Part model, mm, in its own coordinate system. Face numbers are marked on the shaded views. A direction names the side the tool comes from. Round coordinates to 2 decimals unless told otherwise and drop trailing zeros. Loops run counter-clockwise (first coordinate to the right, second up) from the corner with the lowest first, then second, coordinate; pieces in that order, holes last. Notation, with made-up numbers: M 86,84 L 101,84 A15 ccw 101,106 Z; hole C 46,58.25 d2. An arc over 180 degrees is marked long. Answer as CSV lines item,"result". Start each with the question number.
Item 1: Which spindle directions (+Z, -Z, +X, -X, +Y, -Y) get a long thin tool onto all of the face, cutting with end or side? Do the marked faces 1 and 2. Say none if no direction does.
Item 2: Mould opens along X. For the marked faces 3, 4 and 5 say: pulls with the +X half, pulls with the -X half, needs draft (parallel to the pull), parting line crosses it, or undercut.
Item 3: Drop flat-ended pins along their axis: pin 1 Ø2 at (y, z) = (28, -23.5) entering from -X; pin 2 Ø2 at (x, z) = (-12, -23.5) entering from -Y; pin 3 Ø2.5 at (x, y) = (-16, 5) entering from -Z. Give the stop position or say it passes through.
Item 4: Band-saw the part on A-A (x = 0). Give the cut face in (y, z), and give its area (3 significant figures).
Item 5: Band-saw the part on D-D (z = -17). Give the cut face in (x, y).
Item 6: Wall check: line 1 (X direction, y = 53.5, z = -8.5); line 2 (Y direction, x = 5, z = -29.5); line 3 (Z direction, x = -15.55, y = 0). Give the ranges that are in metal, low to high.
Item 7: Band-saw the part on B-B (z = 0). Give the cut face in (x, y).
Item 8: Band-saw the part on C-C (y = 46). Give the cut face in (x, z).
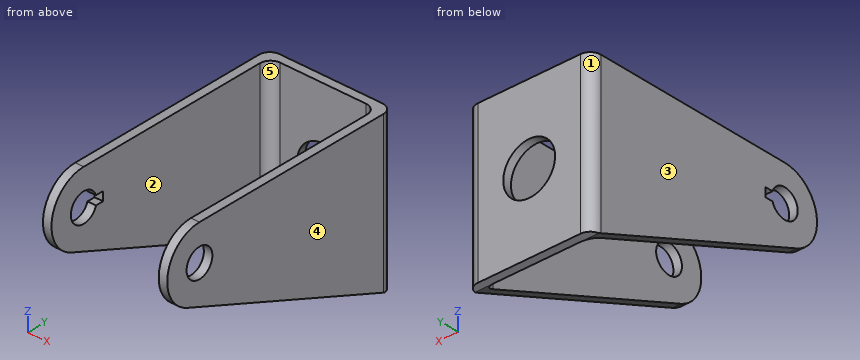
```python
from build123d import *

# Parameters (mm, degrees)
TOP_DEPTH      = 10
TOP_DEPTH_BACK = 34
SKETCH1_W      = 30
SKETCH1_H      = 2.38125
SKETCH2_R      = 10
SKETCH2_R_2    = 4
SKETCH2_W      = 44
SKETCH2_H      = 2.38125
SIDE_DEPTH     = 2.38125
TOP_FILLETS_R  = 3
SKETCH3_R      = 7.25
TOP_HOLE_DEPTH = 80.737744209
KEYWAY_REACH   = 79.23
SKETCH4_W      = 2.5
SKETCH4_H      = 6


with BuildPart() as part:
    # Sketch1 → Top (new, two sides: drawn at the far end of the back side and taken through both)
    with BuildSketch(Plane.XY.offset(-TOP_DEPTH_BACK)):
        with Locations((0, 58.809375)):
            Rectangle(SKETCH1_W, SKETCH1_H)
    extrude(amount=TOP_DEPTH + TOP_DEPTH_BACK)

    # Sketch2 → Side (add)
    # profile 1 of 3: a face of its own
    with BuildSketch(Plane(origin=(15, 0, 0), x_dir=(0, 0, -1), z_dir=(1, 0, 0))):
        with BuildLine():
            Line((34, 57.61875), (-10, 57.61875))
            Line((-10, 57.61875), (-10, 0))
            ThreePointArc((-10, 0), (0, 10), (10, 0))
            ThreePointArc((10, 0), (9.817137723, -1.903629934), (9.275238615, -3.737639447))
            Line((9.275238615, -3.737639447), (34, 57.61875))
        make_face()
    # profile 2 of 3: a face of its own
    with BuildSketch(Plane(origin=(15, 0, 0), x_dir=(0, 0, -1), z_dir=(1, 0, 0))):
        Circle(SKETCH2_R)
        with Locations(Location((0, 0, 0), (0, 0, 180))):
            Circle(SKETCH2_R_2, mode=Mode.SUBTRACT)
    # profile 3 of 3: a face of its own
    with BuildSketch(Plane(origin=(15, 0, 0), x_dir=(0, 0, -1), z_dir=(1, 0, 0))):
        with Locations((12, 58.809375)):
            Rectangle(SKETCH2_W, SKETCH2_H)
    side = extrude(amount=SIDE_DEPTH)

    # Side Mirror: Side across plane
    add(side.mirror(Plane(origin=(0, 0, 0), x_dir=(0, 0, 1), z_dir=(1, 0, 0))))

    # Top Fillets
    top_fillets_edges = [part.edges().sort_by_distance(p)[0] for p in [
        (17.38125, 60, -12),
        (-17.38125, 60, -12),
        (15, 57.61875, -12),
        (-15, 57.61875, -12),
    ]]
    fillet(top_fillets_edges, radius=TOP_FILLETS_R)

    # Sketch3 → Top Hole (cut, through all)
    with BuildSketch(Plane(origin=(0, 60, 0), x_dir=(1, 0, 0), z_dir=(0, 1, 0))):
        with Locations(Location((0, 12, 0), (0, 0, 270))):
            Circle(SKETCH3_R)
    extrude(amount=-TOP_HOLE_DEPTH, mode=Mode.SUBTRACT)

    # Sketch4 → Keyway (cut, up to next)
    with BuildSketch(Plane.ZY.offset(17.38125), mode=Mode.PRIVATE) as keyway_sk1:
        with Locations((0, 3)):
            Rectangle(SKETCH4_W, SKETCH4_H)
    keyway_tool1 = extrude(keyway_sk1.sketch, amount=-KEYWAY_REACH, mode=Mode.PRIVATE) & part.part
    add(keyway_tool1.solids().sort_by_distance((-17.38125, 3, 0))[0], mode=Mode.SUBTRACT)


solid = part.part
```
Answer block:
1,face 1,"+Z, -Z, -X, +Y"
1,face 2,"+Z, -Z, -Y"
2,face 3,"pulls with the -X half"
2,face 4,"pulls with the +X half"
2,face 5,"undercut"
3,pin 1,"passes through"
3,pin 2,"stops at y = 57.45"
3,pin 3,"stops at z = -13.3"
4,outline,"M 57.62,-34 L 60,-34 L 60,-19.25 L 57.62,-19.25 Z; M 57.62,-4.75 L 60,-4.75 L 60,10 L 57.62,10 Z"
4,area,"70.2 mm^2"
5,outline,"M -17.38,15.43 L -15,15.43 L -15,54.62 A3 cw -12,57.62 L -5.25,57.62 L -5.25,60 L -14.38,60 A3 ccw -17.38,57 Z; M 5.25,57.62 L 12,57.62 A3 cw 15,54.62 L 15,15.43 L 17.38,15.43 L 17.38,57 A3 ccw 14.38,60 L 5.25,60 Z"
6,line 1,"x = -17.38 to -15, 15 to 17.38"
6,line 2,"y = 57.62 to 60"
6,line 3,"z = -10.78 to -4, 4 to 10"
7,outline,"M -17.38,-10 L -15,-10 L -15,-4 L -17.38,-4 Z; M -17.38,6 L -15,6 L -15,54.62 A3 cw -12,57.62 L 12,57.62 A3 cw 15,54.62 L 15,4 L 17.38,4 L 17.38,57 A3 ccw 14.38,60 L -14.38,60 A3 ccw -17.38,57 Z; M 15,-10 L 17.38,-10 L 17.38,-4 L 15,-4 Z"
8,outline,"M -17.38,-29.32 L -15,-29.32 L -15,10 L -17.38,10 Z; M 15,-29.32 L 17.38,-29.32 L 17.38,10 L 15,10 Z"
